Read the model definition and answer for the solid it produces. Units are mm, in the model's axes. Coordinates: 2 decimals unless noted, no trailing zeros. Order: outer loops, then holes, each group sorted by start corner. A loop starts at its lowest first (then second) coordinate and runs counter-clockwise, first axis right, second up.
```python
from build123d import *

# Parameters (mm, degrees)
SKETCH1_W           = 25.4
SKETCH1_H           = 124.46
BOSS_EXTRUDE1_DEPTH = 1.27


with BuildPart() as part:
    # Sketch1 → Boss-Extrude1 (new, symmetric)
    with BuildSketch(Plane.XY):
        with Locations((-12.7, -62.23)):
            Rectangle(SKETCH1_W, SKETCH1_H)
        Polygon((50.8, 25.4), (-101.6, 25.4), (-101.6, 0), (-25.4, 0), (0, 0), (50.8, 0), align=None)
    extrude(amount=BOSS_EXTRUDE1_DEPTH, both=True)


solid = part.part
```
1) A cutting plane is placed at C-C, the plane x = -59.5. Determine the outline of the cut face in (y, z), and give its area (3 significant figures).
A:
outline: (0, -1.27) - (25.4, -1.27) - (25.4, 1.27) - (0, 1.27) - close
area: 64.5 mm2
2) A cutting plane is placed at B-B, the plane y = -40.5. Determine the outline of the cut face in (x, z), and give its area (3 significant figures).
A:
outline: (-25.4, -1.27) - (0, -1.27) - (0, 1.27) - (-25.4, 1.27) - close
area: 64.5 mm2
3) Straight lines are drawn through the part: line 1 (X direction, y = -90, z = 0.95); line 2 (Y direction, x = 28, z = 0.5). For each, find the intervals that lie inside material, in ascending order.
A:
line 1: x = -25.4 to 0
line 2: y = 0 to 25.4
4) A cutting plane is placed at A-A, the plane z = -0.05. Determine the outline of the cut face in (x, y).
A:
outline: (-101.6, 0) - (-25.4, 0) - (-25.4, -124.46) - (0, -124.46) - (0, 0) - (50.8, 0) - (50.8, 25.4) - (-101.6, 25.4) - close
